Source: three-view drawing plus pictorial views. Frame: mm from the lowest corner of the part. A direction names the side the tool comes from. Coordinates: 2 decimals unless noted, no trailing zeros. Write each loop counter-clockwise with the first axis right and the second up, starting at its lowest first coordinate (ties: lowest second). Pieces come first, ordered by that corner, then holes. Notation, with made-up numbers: (3.25, 56) - (34.25, 56) arc R29 ccw to (34.25, 86) - close; hole circle Ø6 at (-30, -33). An arc over 180 degrees is marked (long way). Answer as a JSON object with one key per item and string values. Group by question number.
Item 1: Section A-A on x = 95.25. Return loops of the section in (y, z) (1 decimal).
Item 2: Line query: line 1 along Y through (x, z) = (95.25, 0.65) (1 decimal); line 2 along X through (y, z) = (6.5, 1.25); line 3 along Y through (x, z) = (33.5, 11.5). Output: solid intervals per line, ascending. Write a range as from..to.
Item 3: Section B-B on y = 5.08. Return loops of the section in (x, z) (1 decimal).
Item 4: Section D-D on x = 17.5. Return loops of the section in (y, z).
Item 5: First-contact query: pin 1 Ø5.5 at (x, z) = (55, 6.5) entering from -Y; pin 2 Ø3.5 at (x, y) = (65, 5) entering from +Z. Flat tips, straight axial feed; report the tip coordinate or a pass-through.
Item 6: Section C-C on z = 11.5. Return loops of the section in (x, y), and give its area (3 significant figures).
Item 7: Set-up query: the marked faces 1 and 2. Return all of +Z, -Z, +X, -X, +Y, -Y with unobstructed straight access to the full face (end or side cutting, diameter ignored); none if empty.
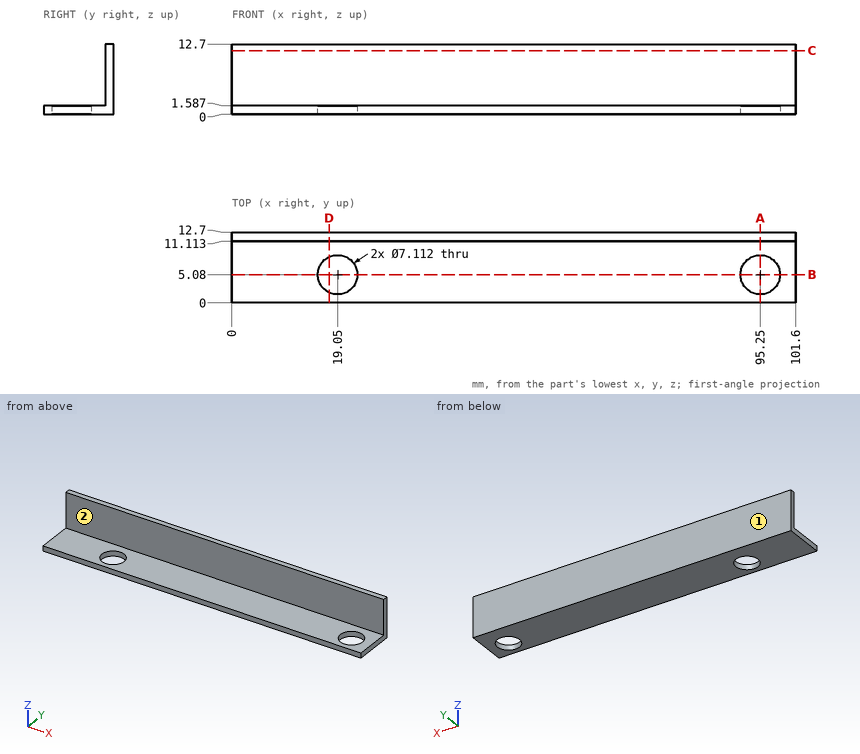
Checks:
{
 "1": {"outline": "(0, 0) - (1.5, 0) - (1.5, 1.6) - (0, 1.6) - close; (8.6, 0) - (12.7, 0) - (12.7, 12.7) - (11.1, 12.7) - (11.1, 1.6) - (8.6, 1.6) - close"},
 "2": {"line 1": "0..1.5, 8.6..12.7", "line 2": "0..15.79, 22.31..91.99, 98.51..101.6", "line 3": "11.11..12.7"},
 "3": {"outline": "(0, 0) - (15.5, 0) - (15.5, 1.6) - (0, 1.6) - close; (22.6, 0) - (91.7, 0) - (91.7, 1.6) - (22.6, 1.6) - close; (98.8, 0) - (101.6, 0) - (101.6, 1.6) - (98.8, 1.6) - close"},
 "4": {"outline": "(0, 0) - (1.88, 0) - (1.88, 1.59) - (0, 1.59) - close; (8.28, 0) - (12.7, 0) - (12.7, 12.7) - (11.11, 12.7) - (11.11, 1.59) - (8.28, 1.59) - close"},
 "5": {"pin 1": "y = 11.11", "pin 2": "z = 1.59"},
 "6": {"outline": "(0, 11.11) - (101.6, 11.11) - (101.6, 12.7) - (0, 12.7) - close", "area": "161 mm^2"},
 "7": {"face 1": "+Z, -Z, +X, -X, +Y", "face 2": "+Z, +X, -X, -Y"}
}
